Work out the finished part from the listing and answer in its coordinate system (mm). Face numbers are marked on the shaded views. A direction names the side the tool comes from. Round coordinates to 2 decimals unless told otherwise and drop trailing zeros. Write each loop counter-clockwise with the first axis right and the second up, starting at its lowest first coordinate (ties: lowest second). Pieces come first, ordered by that corner, then holes.
Autodesk Fusion 360 part; units mm, degrees
sketch "Skizze1" plane through (0, 0, 0) normal (0, 1, 0) x (1, 0, 0)
  line L0 (0, 0) -> (8, 0)
  line L1 (0, 0) -> (0, -12)
  line L2 (8, 0) -> (8, -12)
  line L3 (0, -12) -> (8, -12)
  dimension "d1" = 8
  dimension "d2" = 12
  dimension "d3" = 12
extrude "Extrusion1" add sketch "Skizze1" along normal blind 4
sketch "Skizze2" plane through (0, 4, 0) normal (0, 1, 0) x (-1, 0, 0)
  line L0 (0, 0) -> (0, 12)
  line L1 (0, 12) -> (-8, 12)
  line L2 (-8, 12) -> (-8, 0)
  line L3 (-8, 0) -> (0, 0)
  circle A0 centre (-4, 5) radius 1.5
  dimension "d6" = 3
extrude "Extrusion2" cut sketch "Skizze2" against normal blind 15 contours A0
sketch "Skizze3" plane through (0, 4, 0) normal (0, 1, 0) x (-1, 0, 0)
  circle A0 centre (-4, 5) radius 1.5
  line L0 (0, 0) -> (0, 12)
  line L1 (0, 12) -> (-8, 12)
  line L2 (-8, 12) -> (-8, 0)
  line L3 (-8, 0) -> (0, 0)
  line L4 (0, 12) -> (0, 9)
  line L5 (0, 9) -> (0, 8)
  line L6 (0, 8) -> (-8, 8)
  line L7 (-8, 8) -> (-8, 12)
  line L8 (-8, 12) -> (0, 12)
extrude "Extrusion3" add sketch "Skizze3" along normal blind 30 contours L0 L1 L2 L4 L5 L6 L7 L8
sketch "Skizze4" plane through (0, 0, 12) normal (0, 0, 1) x (1, 0, 0)
  line L0 (0, 0) -> (8, 0)
  line L1 (8, 0) -> (8, 34)
  line L2 (8, 34) -> (0, 34)
  line L3 (0, 34) -> (0, 0)
  line L4 (0, 34) -> (0, 29)
  line L5 (0, 29) -> (4, 29)
  circle A0 centre (4, 29) radius 1.5
  dimension "d11" = 3
extrude "Extrusion4" cut sketch "Skizze4" against normal blind 21 contours A0
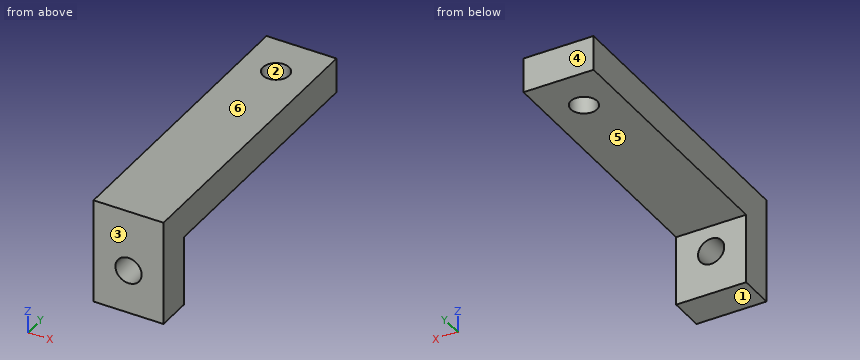
Q1. Find the intervals of material crossed by L1, parallel to Y at x = 4, z = 9.35; L2, parallel to Z at x = 4, y = 1.55; L3, parallel to Y at x = 5, z = 3.75, in increasing order.
Q2. Find section D-D (z = 8.5). Determine the outline of the cut face in (x, y).
Q3. Given pin 1 (4 mm diameter, centred on x = 7, z = 5.5, fed in from +Y), flat-ended and moving along its own axis, determine where the tip first touches the part or whether it passes through.
Q4. Find section B-B (z = 5). Determine the outline of the cut face in (x, y), plus the area to 3 significant figures.
Q5. The mould has two halves that part along Y. Classify the marked faces 1, 2, 3 and 4: +Y half, -Y half, draft (parallel to the pull), parting line (faces both ways), or undercut.
Q6. Find section C-C (x = 4). Determine the outline of the cut face in (y, z), plus the area to 3 significant figures.
Q7. Find section A-A (y = 29). Determine the outline of the cut face in (x, z).
Q8. A tool of negligible diameter and unlimited length cuts with its end or side. For the marked faces 5 and 6, from which of +Z, -Z, +X, -X, +Y, -Y can it reach the whole face along a straight path? Write none if from no direction.
Report:
1. L1: y = 0 to 27.5, 30.5 to 34
1. L2: z = 0 to 3.5, 6.5 to 12
1. L3: y = 0 to 4
2. outline: (0, 0) - (8, 0) - (8, 34) - (0, 34) - close; hole circle Ø3 at (4, 29)
3. pin 1: stops at y = 4
4. outline: (0, 0) - (2.5, 0) - (2.5, 4) - (0, 4) - close; (5.5, 0) - (8, 0) - (8, 4) - (5.5, 4) - close
4. area: 20.0 mm2
5. face 1: draft
5. face 2: undercut
5. face 3: -Y half
5. face 4: +Y half
6. outline: (0, 0) - (4, 0) - (4, 3.5) - (0, 3.5) - close; (0, 6.5) - (4, 6.5) - (4, 8) - (27.5, 8) - (27.5, 12) - (0, 12) - close; (30.5, 8) - (34, 8) - (34, 12) - (30.5, 12) - close
6. area: 144 mm2
7. outline: (0, 8) - (2.5, 8) - (2.5, 12) - (0, 12) - close; (5.5, 8) - (8, 8) - (8, 12) - (5.5, 12) - close
8. face 5: -Z, +X, -X, +Y
8. face 6: +Z, +X, -X, +Y, -Y
